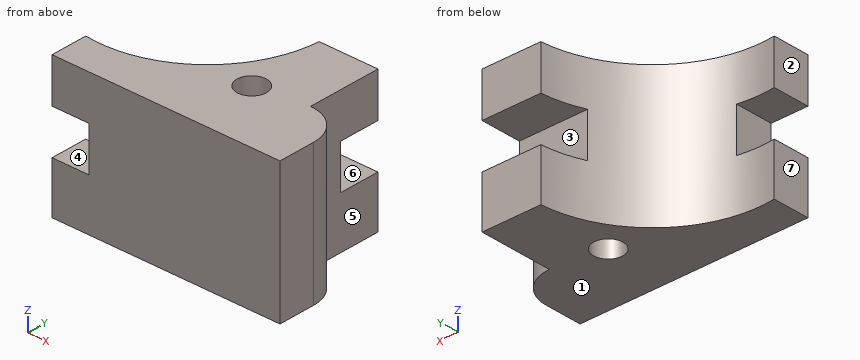
from build123d import *

# Parameters (mm, degrees)
BOSS_EXTRUDE1_DEPTH = 60.325
SKETCH2_W           = 19.05
SKETCH2_H           = 17.526
CUT_EXTRUDE1_DEPTH  = 29.8196
SKETCH3_W           = 15.875
SKETCH3_H           = 19.05
CUT_EXTRUDE2_DEPTH  = 29.8196
SKETCH4_R           = 6.35
CUT_EXTRUDE3_DEPTH  = 60.3504


with BuildPart() as part:
    # Sketch1 → Boss-Extrude1 (new body)
    with BuildSketch(Plane.XY):
        with BuildLine():
            Line((0, 0), (82.55, 0))
            Line((82.55, 0), (98.425, 0))
            Line((98.425, 0), (98.425, 15.9004))
            ThreePointArc((98.425, 15.9004), (93.782759639, 27.107759639), (82.5754, 31.75))
            Line((82.5754, 31.75), (82.55, 31.75))
            Line((82.55, 31.75), (82.55, 63.5))
            Line((82.55, 63.5), (57.15, 63.5))
            ThreePointArc((57.15, 63.5), (38.947337741, 27.240694711), (0, 15.875))
            Line((0, 15.875), (0, 0))
        make_face()
    extrude(amount=-BOSS_EXTRUDE1_DEPTH)

    # Sketch2 → Cut-Extrude1 (cut)
    with BuildSketch(Plane(origin=(82.55, 0, 0), x_dir=(0, 0, -1), z_dir=(1, 0, 0))):
        with Locations((28.575, 54.737)):
            Rectangle(SKETCH2_W, SKETCH2_H)
    extrude(amount=-CUT_EXTRUDE1_DEPTH, mode=Mode.SUBTRACT)

    # Sketch3 → Cut-Extrude2 (cut)
    with BuildSketch(Plane.XZ):
        with Locations((7.9375, -28.575)):
            Rectangle(SKETCH3_W, SKETCH3_H)
    extrude(amount=-CUT_EXTRUDE2_DEPTH, mode=Mode.SUBTRACT)

    # Sketch4 → Cut-Extrude3 (cut)
    with BuildSketch(Plane.XY):
        with Locations((60.071, 28.575)):
            Circle(SKETCH4_R)
    extrude(amount=-CUT_EXTRUDE3_DEPTH, mode=Mode.SUBTRACT)


solid = part.part
The model under review builds one solid part; all positions refer to its coordinate system, in mm. Face numbers are marked on the shaded views. A direction names the side the tool comes from. Give positions to 0.01 mm unless a question says otherwise; leave off trailing zeros. Loops run counter-clockwise (first coordinate to the right, second up) from the corner with the lowest first, then second, coordinate; pieces in that order, holes last. Notation, with made-up numbers: (32, 68.5) -> (60, 68.5) arc R33 ccw to (60, 97.5) -> close; hole circle Ø3 at (76.5, 51.5). An arc over 180 degrees is marked (long way). Answer as a JSON object with one key per item and string values. Group by question number.
Q1. Draft analysis for pull direction Z (two halves, no side actions). For the marked faces 1, 2 and 3, state which applies: pulls with the +Z half, pulls with the -Z half, needs draft (parallel to the pull), parting line crosses it, or undercut.
Q2. Tool access review of the marked faces 4, 5, 6 and 7: name each direction out of +Z, -Z, +X, -X, +Y, -Y from which nothing blocks a thin tool from reaching the whole face with its end or side.
Q3. Take a section at A-A (y = 53.5). Write out the cut boundary in (x, z) (3 decimals), plus the area to 3 significant figures.
Q4. Take a section at B-B (z = -32). Write out the cut boundary in (x, y) (3 decimals).
Q5. Insertion check: pin 1 (1 mm diameter, centred on y = 47, z = -14, fed in from +X); pin 2 (12 mm diameter, centred on x = 36.5, z = -50, fed in from +Y); pin 3 (8 mm diameter, centred on y = 10, z = -29.5, fed in from -X) (3 decimals). Each pin has a flat end and moves straight along its axis. Give the tip position at first contact, or say it passes through.
Q6. Wall thickness on line 1 along Z through (x, y) = (14, 12) (3 decimals); line 2 along Y through (x, z) = (59, -43); line 3 along X through (y, z) = (26.5, -22): over which ranges is each line inside the solid? List them lowest first.
Q7. Take a section at C-C (y = 13.5). Write out the cut boundary in (x, z) (3 decimals), plus the area to 3 significant figures.
Q8. Take a section at D-D (x = 78.5). Write out the cut boundary in (y, z) (3 decimals).
Answer below:
{
 "1": {"face 1": "pulls with the -Z half", "face 2": "needs draft", "face 3": "undercut"},
 "2": {"face 4": "-X, +Y, -Y", "face 5": "+Z, -Z, +X, +Y", "face 6": "+X, -X, +Y", "face 7": "+Z, -Z, -X, +Y, -Y"},
 "3": {"outline": "(55.595, -60.325) -> (82.55, -60.325) -> (82.55, -38.1) -> (55.595, -38.1) -> close; (55.595, -19.05) -> (82.55, -19.05) -> (82.55, 0) -> (55.595, 0) -> close", "area": "1,110 mm2"},
 "4": {"outline": "(15.875, 0) -> (98.425, 0) -> (98.425, 15.9) arc R15.85 ccw to (82.575, 31.75) -> (82.55, 31.75) -> (82.55, 45.974) -> (52.997, 45.974) arc R50.798 cw to (15.875, 16.353) -> close; hole circle Ø12.7 at (60.071, 28.575)"},
 "5": {"pin 1": "stops at x = 82.55", "pin 2": "stops at y = 30.5", "pin 3": "stops at x = 15.875"},
 "6": {"line 1": "z = -60.325 to -38.1, -19.05 to 0", "line 2": "y = 0 to 22.32, 34.83 to 63.5", "line 3": "x = 38.04 to 54.07, 66.07 to 94.36"},
 "7": {"outline": "(0, -60.325) -> (98.425, -60.325) -> (98.425, 0) -> (0, 0) -> (0, -19.05) -> (15.875, -19.05) -> (15.875, -38.1) -> (0, -38.1) -> close", "area": "5,640 mm2"},
 "8": {"outline": "(0, -60.325) -> (63.5, -60.325) -> (63.5, -38.1) -> (45.974, -38.1) -> (45.974, -19.05) -> (63.5, -19.05) -> (63.5, 0) -> (0, 0) -> close"}
}
